from build123d import *

# Parameters (mm, degrees)
BOSS_EXTRUDE1_DEPTH = 10
SKETCH2_R           = 1.25
CUT_EXTRUDE1_DEPTH  = 40.220402854
CUT_EXTRUDE2_REACH  = 39.524
SKETCH3_R           = 2.5
FILLET1_R           = 0.5
FILLET2_R           = 5


with BuildPart() as part:
    # Sketch1 → Boss-Extrude1 (new body)
    with BuildSketch(Plane.XY):
        Polygon((0, 0), (8, 0), (8, -20.2), (30, -20.2), (30, -23.2), (5, -23.2), (5, -9), (0, -9), (0, -6), (5, -6), (5, -3), (0, -3), align=None)
    extrude(amount=BOSS_EXTRUDE1_DEPTH)

    # Sketch2 → Cut-Extrude1 (cut, through all)
    with BuildSketch(Plane(origin=(0, 0, 0), x_dir=(1, 0, 0), z_dir=(0, 1, 0))):
        with Locations(Location((2.28, -5, 0), (0, 0, 270))):
            Circle(SKETCH2_R)
    extrude(amount=-CUT_EXTRUDE1_DEPTH, mode=Mode.SUBTRACT)

    # Sketch3 → Cut-Extrude2 (cut, up to next)
    with BuildSketch(Plane(origin=(0, -20.2, 0), x_dir=(1, 0, 0), z_dir=(0, 1, 0)), mode=Mode.PRIVATE) as cut_extrude2_sk1:
        with Locations(Location((25, -5, 0), (0, 0, 270))):
            Circle(SKETCH3_R)
    cut_extrude2_tool1 = extrude(cut_extrude2_sk1.sketch, amount=-CUT_EXTRUDE2_REACH, mode=Mode.PRIVATE) & part.part
    # Sketch3 → Cut-Extrude2 (cut, up to next)
    with BuildSketch(Plane(origin=(0, -20.2, 0), x_dir=(1, 0, 0), z_dir=(0, 1, 0)), mode=Mode.PRIVATE) as cut_extrude2_sk2:
        with Locations(Location((15, -5, 0), (0, 0, 270))):
            Circle(SKETCH3_R)
    cut_extrude2_tool2 = extrude(cut_extrude2_sk2.sketch, amount=-CUT_EXTRUDE2_REACH, mode=Mode.PRIVATE) & part.part
    add(cut_extrude2_tool1.solids().sort_by_distance((25, -20.2, 5))[0], mode=Mode.SUBTRACT)
    add(cut_extrude2_tool2.solids().sort_by_distance((15, -20.2, 5))[0], mode=Mode.SUBTRACT)

    # Fillet1
    fillet1_edges = [part.edges().sort_by_distance(p)[0] for p in [
        (4, 0, 0),
        (8, -10.1, 0),
        (5, -4.5, 10),
        (19, -20.2, 0),
        (17.5, -23.2, 0),
        (5, -16.1, 0),
        (2.5, -9, 0),
        (0, -7.5, 0),
        (2.5, -6, 0),
        (5, -4.5, 0),
        (2.5, -3, 0),
        (0, -1.5, 0),
        (2.5, -6, 10),
        (0, 0, 5),
        (8, 0, 5),
        (8, -20.2, 5),
        (0, -7.5, 10),
        (30, -20.2, 5),
        (30, -23.2, 5),
        (5, -23.2, 5),
        (5, -9, 5),
        (0, -9, 5),
        (2.5, -9, 10),
        (5, -16.1, 10),
        (17.5, -23.2, 10),
        (19, -20.2, 10),
        (8, -10.1, 10),
        (4, 0, 10),
        (0, -1.5, 10),
        (2.5, -3, 10),
    ]]
    fillet(fillet1_edges, radius=FILLET1_R)

    # Fillet2
    # the kernel refuses this fillet: 5 mm, written as the material it takes off along each edge
    with BuildSketch(Plane(origin=(25, -20.2, 5), x_dir=(1, 0, 0), z_dir=(0, 0, 1))) as fillet2_piece_1:
        with BuildLine():
            CenterArc((4.5, -0.5), 0.5, 0, 90)
            Line((5, -0.5), (5, 0))
            Line((5, 0), (4.5, 0))
        make_face()
    revolve(axis=Axis((25, -20.2, 5), (0, 1, 0)), revolution_arc=90, mode=Mode.SUBTRACT)
    with BuildSketch(Plane(origin=(25, -23.2, 5), x_dir=(0, 0, -1), z_dir=(-1, 0, 0))) as fillet2_piece_2:
        with BuildLine():
            CenterArc((4.5, -0.5), 0.5, 0, 90)
            Line((5, -0.5), (5, 0))
            Line((5, 0), (4.5, 0))
        make_face()
    revolve(axis=Axis((25, -23.2, 5), (0, -1, 0)), revolution_arc=90, mode=Mode.SUBTRACT)
    with BuildSketch(Plane(origin=(25, -20.2, 5), x_dir=(0, 0, 1), z_dir=(-1, 0, 0))) as fillet2_piece_3:
        with BuildLine():
            CenterArc((4.5, -0.5), 0.5, 0, 90)
            Line((5, -0.5), (5, 0))
            Line((5, 0), (4.5, 0))
        make_face()
    revolve(axis=Axis((25, -20.2, 5), (0, 1, 0)), revolution_arc=90, mode=Mode.SUBTRACT)
    with BuildSketch(Plane(origin=(25, -23.2, 5), x_dir=(1, 0, 0), z_dir=(0, 0, -1))) as fillet2_piece_4:
        with BuildLine():
            CenterArc((4.5, -0.5), 0.5, 0, 90)
            Line((5, -0.5), (5, 0))
            Line((5, 0), (4.5, 0))
        make_face()
    revolve(axis=Axis((25, -23.2, 5), (0, -1, 0)), revolution_arc=90, mode=Mode.SUBTRACT)
    with BuildSketch(Plane(origin=(30, -20.2, 10), x_dir=(-1, 0, 0), z_dir=(0, -1, 0))) as fillet2_piece_5:
        with BuildLine():
            CenterArc((FILLET2_R, FILLET2_R), FILLET2_R, 180, 90)
            Line((0, FILLET2_R), (0, 0))
            Line((0, 0), (FILLET2_R, 0))
        make_face()
    extrude(amount=3, mode=Mode.SUBTRACT)
    with BuildSketch(Plane(origin=(30, -20.2, 0), x_dir=(-1, 0, 0), z_dir=(0, -1, 0))) as fillet2_piece_6:
        with BuildLine():
            CenterArc((FILLET2_R, -FILLET2_R), FILLET2_R, 90, 90)
            Line((0, -FILLET2_R), (0, 0))
            Line((0, 0), (FILLET2_R, 0))
        make_face()
    extrude(amount=3, mode=Mode.SUBTRACT)


solid = part.part
Build history of the part. All positions in model axes, mm. A direction names the side the tool comes from. Round coordinates to 2 decimals unless told otherwise and drop trailing zeros. Loops run counter-clockwise (first coordinate to the right, second up) from the corner with the lowest first, then second, coordinate; pieces in that order, holes last. Notation, with made-up numbers: (45, -1.5) -> (90, -1.5) arc R20 ccw to (90, 4.5) -> close; hole circle Ø3 at (9.25, 66.25). An arc over 180 degrees is marked (long way). Use CSV: the item, a comma, the result in double quotes. Start each with the question number.
Q1. Mould opens along Y. For faces 1 (the face through (4, -9, 5)), 2 (the face through (12.78, -21.68, 6.15)), 3 (the face through (4, -6, 5)) say: +Y half, -Y half, draft (parallel to the pull), parting line (faces both ways), or undercut.
Q2. Saw through at D-D on z = 5. Count the separate pieces of the cut face and the enclosed holes in it, and give its area (3 significant figures).
Q3. Drill centre lines: L1, parallel to X at y = -21.1, z = 5; L2, parallel to X at y = -22, z = 6; L3, parallel to X at y = -0.75, z = 9. Where is each one in solid material? Low to high.
Q4. Saw through at C-C on y = -1.75. Give the cut face in (x, z).
Q5. Saw through at B-B on x = 15. Give the cut face in (y, z), and give its area (3 significant figures).
Q6. Which spindle directions (+Z, -Z, +X, -X, +Y, -Y) get a long thin tool onto all of the face, cutting with end or side? Do faces 4 (the face through (19, -20.2, 5)), 5 (the face through (5, -16, 5)), 6 (the face through (4, -3, 5)). Say none if no direction does.
Q7. Saw through at A-A on x = 2.28. Give the cut face in (y, z), and give its area (3 significant figures).
Q8. Flat gauge pins, fed straight in: pin 1 Ø3.5 at (y, z) = (-4, 6) entering from -X; pin 2 Ø6 at (y, z) = (-19.5, 1) entering from +X; pin 3 Ø5 at (y, z) = (-11, 6.5) entering from +X; pin 4 Ø4 at (y, z) = (-14.5, 6) entering from -X. Where does each tip first touch, or does it go through?
Solutions:
1,face 1,"-Y half"
1,face 2,"draft"
1,face 3,"undercut"
2,separate pieces,"5"
2,enclosed holes,"0"
2,area,"120 mm^2"
3,L1,"x = 5 to 12.5, 17.5 to 22.5, 27.5 to 30"
3,L2,"x = 5 to 12.71, 17.29 to 22.71, 27.29 to 29.9"
3,L3,"x = 0 to 8"
4,outline,"(0, 0.5) arc R0.5 ccw to (0.5, 0) -> (7.5, 0) arc R0.5 ccw to (8, 0.5) -> (8, 9.5) arc R0.5 ccw to (7.5, 10) -> (0.5, 10) arc R0.5 ccw to (0, 9.5) -> close; hole circle Ø2.5 at (2.28, 5)"
5,outline,"(-23.2, 0.5) arc R0.5 ccw to (-22.7, 0) -> (-20.7, 0) arc R0.5 ccw to (-20.2, 0.5) -> (-20.2, 2.5) -> (-23.2, 2.5) -> close; (-23.2, 7.5) -> (-20.2, 7.5) -> (-20.2, 9.5) arc R0.5 ccw to (-20.7, 10) -> (-22.7, 10) arc R0.5 ccw to (-23.2, 9.5) -> close"
5,area,"14.8 mm^2"
6,face 4,"+Z, -Z, +X, +Y"
6,face 5,"+Z, -Z, -X, -Y"
6,face 6,"+Z, -Z, -X"
7,outline,"(-9, 0.5) arc R0.5 ccw to (-8.5, 0) -> (-6.5, 0) arc R0.5 ccw to (-6, 0.5) -> (-6, 3.75) -> (-9, 3.75) -> close; (-9, 6.25) -> (-6, 6.25) -> (-6, 9.5) arc R0.5 ccw to (-6.5, 10) -> (-8.5, 10) arc R0.5 ccw to (-9, 9.5) -> close; (-3, 0.5) arc R0.5 ccw to (-2.5, 0) -> (-0.5, 0) arc R0.5 ccw to (0, 0.5) -> (0, 3.75) -> (-3, 3.75) -> close; (-3, 6.25) -> (0, 6.25) -> (0, 9.5) arc R0.5 ccw to (-0.5, 10) -> (-2.5, 10) arc R0.5 ccw to (-3, 9.5) -> close"
7,area,"44.6 mm^2"
8,pin 1,"stops at x = 0"
8,pin 2,"stops at x = 29.84"
8,pin 3,"stops at x = 8"
8,pin 4,"stops at x = 5"
